The listing builds one solid part. Answer for the finished solid, in the listing's coordinates (mm). A direction names the side the tool comes from. Coordinates: 2 decimals unless noted, no trailing zeros. Order: outer loops, then holes, each group sorted by start corner. A loop starts at its lowest first (then second) coordinate and runs counter-clockwise, first axis right, second up. Notation, with made-up numbers: (25.25, 40) -> (72.25, 40) arc R29 ccw to (72.25, 78) -> close; hole circle Ø6 at (89.5, -11). An arc over 180 degrees is marked (long way). Put each result on its own line as item: value. Start each with the question number.
```python
from build123d import *

# Parameters (mm, degrees)
BOSS_EXTRUDE1_DEPTH = 40.2
SKETCH2_W           = 31.8
SKETCH2_H           = 38.8
BOSS_EXTRUDE2_DEPTH = 12.6
FILLET1_R           = 3
FILLET2_R           = 3
FILLET3_R           = 2


with BuildPart() as part:
    # Sketch1 → Boss-Extrude1 (new body)
    with BuildSketch(Plane(origin=(0, 0, 0), x_dir=(0, 0, -1), z_dir=(1, 0, 0))):
        Polygon((46.15, 0), (-46.15, 0), (-46.15, 11.3), (9.024430632, 11.3), (13.351719093, 14.33), (28.351719093, 14.33), (34.15, 18.39), (46.15, 18.39), align=None)
    extrude(amount=-BOSS_EXTRUDE1_DEPTH)

    # Sketch2 → Boss-Extrude2 (add)
    with BuildSketch(Plane(origin=(0, 11.3, 0), x_dir=(1, 0, 0), z_dir=(0, 1, 0))):
        with Locations((-20.1, -4.375569368)):
            Rectangle(SKETCH2_W, SKETCH2_H)
    extrude(amount=BOSS_EXTRUDE2_DEPTH)

    # Fillet1
    fillet1_edges = [part.edges().sort_by_distance(p)[0] for p in [
        (-36, 19.115, -15.024430632),
        (-4.2, 19.115, -15.024430632),
        (-36, 17.6, 23.775569368),
        (-4.2, 17.6, 23.775569368),
    ]]
    fillet(fillet1_edges, radius=FILLET1_R)

    # Fillet2
    fillet2_edges = [part.edges().sort_by_distance(p)[0] for p in [
        (0, 9.195, -46.15),
        (0, 5.65, 46.15),
        (-40.2, 9.195, -46.15),
        (-40.2, 5.65, 46.15),
    ]]
    fillet(fillet2_edges, radius=FILLET2_R)

    # Fillet3
    fillet3_edges = [part.edges().sort_by_distance(p)[0] for p in [
        (-38.1, 11.3, -9.024430632),
        (-2.1, 11.3, -9.024430632),
        (-37.945204942, 14.33, -13.351719093),
        (-2.254795058, 14.33, -13.351719093),
        (-20.1, 14.33, -28.351719093),
        (-20.1, 18.39, -34.15),
    ]]
    fillet(fillet3_edges, radius=FILLET3_R)


solid = part.part
```
(1) Each of these flat-tipped pins is pushed along its axis until it touches: P1, Ø5, axis at x = -26.5, z = 37, coming from the +Y side; P2, Ø9, axis at x = -17.5, z = -40.5, coming from the +Y side; P3, Ø4, axis at x = -27.5, z = -18.5, coming from the +Y side. Where does it stop, or does it pass through?
(2) The part is cut by section A-A on z = 0.5. Determine the outline of the cut face in (x, y), plus the area to 3 significant figures.
(3) Find the intervals of material crossed by L1, parallel to Z at x = -25, y = 18.5; L2, parallel to Z at x = -12, y = 16.5; L3, parallel to Y at x = -21.5, z = 40, in increasing order.
(4) A tool of negligible diameter and unlimited length cuts with its end or side. For faces 5 (the flat face through (-36, 18, 5)), 6 (the flat face through (-20, 6, 46.15)), 7 (the cylindrical face through (-39.34, 9.07, -45.25)), 8 (the flat face through (-19.82, 16.34, -31.22)), 9 (the flat face through (-20, 18.39, -40)), from which of +Z, -Z, +X, -X, +Y, -Y can it reach the whole face along a straight path? Write none if from no direction.
(5) The part is cut by section B-B on y = 16.25. Determine the outline of the cut face in (x, z).
(6) The part is cut by section C-C on y = 22. Determine the outline of the cut face in (x, z), plus the area to 3 significant figures.
(7) The part is cut by section D-D on x = -26.5. Determine the outline of the cut face in (y, z), plus the area to 3 significant figures.
(8) For a pull along Z with two mould halves and no side action, classify faces 1 (the cylindrical face through (-0.86, 9.07, -45.25)), 2 (the cylindrical face through (-5.102, 18.724, -14.169)), 3 (the cylindrical face through (-35.145, 17.688, 22.873)), 4 (the flat face through (-4.2, 18, 5)) as released by +Z, released by -Z, zero draft, split by the parting line, or undercut.
Worked out:
1. P1: y = 11.3
1. P2: y = 18.39
1. P3: y = 14.33
2. outline: (-40.2, 0) -> (0, 0) -> (0, 11.3) -> (-4.2, 11.3) -> (-4.2, 23.9) -> (-36, 23.9) -> (-36, 11.3) -> (-40.2, 11.3) -> close
2. area: 855 mm2
3. L1: -15.02 to 23.78
3. L2: -46.15 to -31.45, -15.02 to 23.78
3. L3: 0 to 11.3
4. face 5: +Z, -X, +Y
4. face 6: +Z, +X, -X, +Y, -Y
4. face 7: -Z, -X, +Y, -Y
4. face 8: +X, -X, +Y
4. face 9: -Z, +X, -X, +Y
5. outline: (-40.2, -43.15) arc R3 ccw to (-37.2, -46.15) -> (-3, -46.15) arc R3 ccw to (0, -43.15) -> (0, -31.09) -> (-40.2, -31.09) -> close; (-36, -12.02) arc R3 ccw to (-33, -15.02) -> (-7.2, -15.02) arc R3 ccw to (-4.2, -12.02) -> (-4.2, 20.78) arc R3 ccw to (-7.2, 23.78) -> (-33, 23.78) arc R3 ccw to (-36, 20.78) -> close
6. outline: (-36, -12.02) arc R3 ccw to (-33, -15.02) -> (-7.2, -15.02) arc R3 ccw to (-4.2, -12.02) -> (-4.2, 20.78) arc R3 ccw to (-7.2, 23.78) -> (-33, 23.78) arc R3 ccw to (-36, 20.78) -> close
6. area: 1,230 mm2
7. outline: (0, -46.15) -> (18.39, -46.15) -> (18.39, -34.78) arc R2 ccw to (18.03, -33.63) -> (14.69, -28.87) arc R2 cw to (14.33, -27.72) -> (14.33, -15.02) -> (23.9, -15.02) -> (23.9, 23.78) -> (11.3, 23.78) -> (11.3, 46.15) -> (0, 46.15) -> close
7. area: 1,690 mm2
8. face 1: released by -Z
8. face 2: undercut
8. face 3: released by +Z
8. face 4: zero draft
